Source: three-view drawing plus pictorial views. Frame: mm from the lowest corner of the part. A direction names the side the tool comes from. Give positions to 0.01 mm unless a question says otherwise; leave off trailing zeros. Order: outer loops, then holes, each group sorted by start corner. A loop starts at its lowest first (then second) coordinate and runs counter-clockwise, first axis right, second up.
1) Material intervals for line 1 (X direction, y = 12.05, z = 2.35); line 2 (X direction, y = 13.35, z = 17.65); line 3 (Z direction, x = 16.1, y = 13.15), sorted ascending.
2) Section C-C, the plane x = 44.6. Return loops of the section in (y, z), plus the area to 3 significant figures.
3) Section A-A, the plane y = 5. Return loops of the section in (x, z).
4) Section B-B, the plane z = 17.65. Return loops of the section in (x, y).
5) Access query for the marked faces 1 and 2. Directions: +Z, -Z, +X, -X, +Y, -Y. A direction counts if a zero-diameter tool reaches every point of the face in a straight line with its end or side. Return the directions, or none.
6) Section D-D, the plane z = 13.25. Return loops of the section in (x, y).
7) First-contact query: P1, Ø3, axis at x = 42, z = 17.65, coming from the +Y side; P2, Ø2, axis at y = 8.5, z = 10, coming from the -X side; P3, Ø3.5, axis at y = 5, z = 6, coming from the +X side; P4, Ø6, axis at x = 43.5, z = 4, coming from the -Y side. Flat tips, straight axial feed; report the tip coordinate or a pass-through.
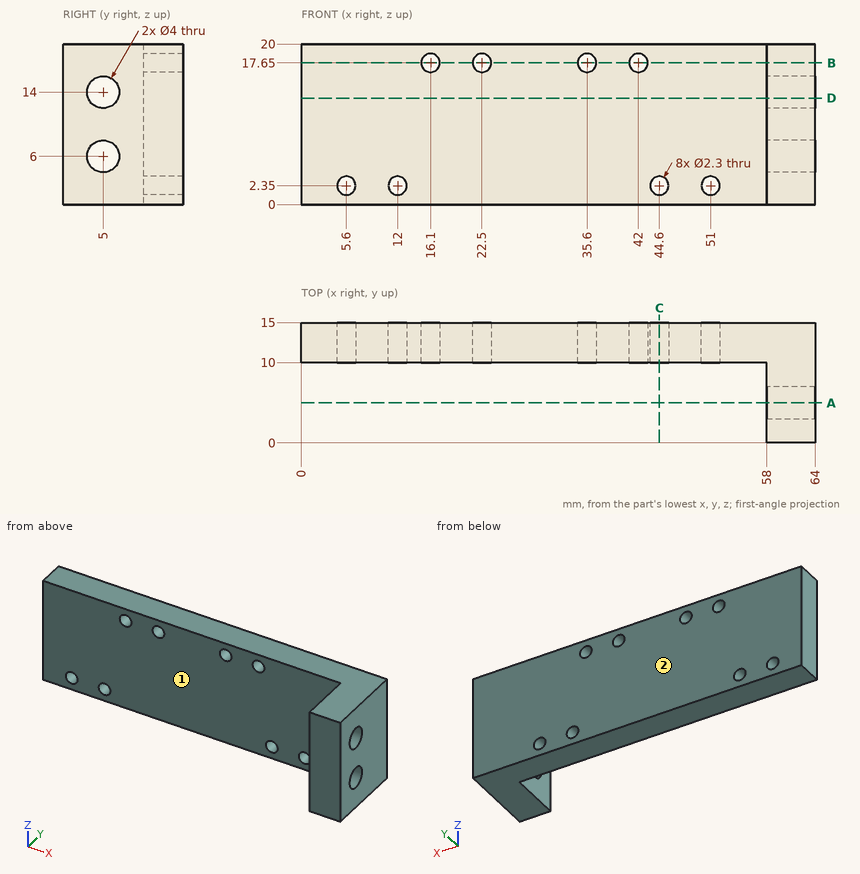
From the geometry:
1. line 1: x = 0 to 4.45, 6.75 to 10.85, 13.15 to 43.45, 45.75 to 49.85, 52.15 to 64
1. line 2: x = 0 to 14.95, 17.25 to 21.35, 23.65 to 34.45, 36.75 to 40.85, 43.15 to 64
1. line 3: z = 0 to 16.5, 18.8 to 20
2. outline: (10, 0) - (15, 0) - (15, 1.2) - (10, 1.2) - close; (10, 3.5) - (15, 3.5) - (15, 20) - (10, 20) - close
2. area: 88.5 mm2
3. outline: (58, 0) - (64, 0) - (64, 4) - (58, 4) - close; (58, 8) - (64, 8) - (64, 12) - (58, 12) - close; (58, 16) - (64, 16) - (64, 20) - (58, 20) - close
4. outline: (0, 10) - (14.95, 10) - (14.95, 15) - (0, 15) - close; (17.25, 10) - (21.35, 10) - (21.35, 15) - (17.25, 15) - close; (23.65, 10) - (34.45, 10) - (34.45, 15) - (23.65, 15) - close; (36.75, 10) - (40.85, 10) - (40.85, 15) - (36.75, 15) - close; (43.15, 10) - (58, 10) - (58, 0) - (64, 0) - (64, 15) - (43.15, 15) - close
5. face 1: +Z, -Z, -X, -Y
5. face 2: +Z, -Z, +X, -X, +Y
6. outline: (0, 10) - (58, 10) - (58, 6.85) - (64, 6.85) - (64, 15) - (0, 15) - close; (58, 0) - (64, 0) - (64, 3.15) - (58, 3.15) - close
7. P1: stops at y = 15
7. P2: stops at x = 58
7. P3: passes through
7. P4: stops at y = 10
